Verification items for the finished model (mm, model axes). A direction names the side the tool comes from. Give positions to 0.01 mm unless a question says otherwise; leave off trailing zeros. Write each loop counter-clockwise with the first axis right and the second up, starting at its lowest first coordinate (ties: lowest second). Pieces come first, ordered by that corner, then holes. Notation, with made-up numbers: (21.25, 18.5) - (47.25, 18.5) arc R37 cw to (47.25, 56.5) - close; hole circle Ø6 at (55.25, 67.5). An arc over 180 degrees is marked (long way). Answer as a JSON object with one key per item and string values. Group by question number.
Item 1: Sectioned sample at B-B, the plane x = 0.95. Count the separate pieces of the cut face and the enclosed holes in it, and give its area (3 significant figures).
Item 2: Scan lines: line 1 along Y through (x, z) = (2.3, 0); line 2 along Y through (x, z) = (1.9, 16.5); line 3 along Z through (x, y) = (0.3, 16). Record each from-to range of solid material in increasing order. Write a range as [from, to].
Item 3: Tool access check on faces 1 (the face through (1, -17.1, -15)), 2 (the face through (1, -25, -23)), 3 (the face through (1, -25, 19)), 4 (the face through (2, 32, -35)). Record the directions out of +Z, -Z, +X, -X, +Y, -Y that give a thin tool (end or side, any length) a straight path to the whole face; none if there is none.
Item 4: Sectioned sample at C-C, the plane y = -7.5. Record the boundary of the cut face in (x, z).
Item 5: Sectioned sample at A-A, the plane y = 16. Record the boundary of the cut face in (x, z).
Item 6: Sectioned sample at D-D, the plane z = -20. Record the boundary of the cut face in (x, y).
Item 7: Go/stop test with flat-tipped pins: pin 1 (2 mm diameter, centred on y = -20.5, z = -46.5, fed in from -X); pin 2 (1.5 mm diameter, centred on x = 1.5, z = 16, fed in from -Y); pin 3 (1.5 mm diameter, centred on x = 1.5, y = -16, fed in from -Z); pin 4 (0.9 mm diameter, centred on x = 2, y = 31.5, fed in from -Z). Record where each tip stops, or that it passes through.
Item 8: Draft check along Y on faces 5 (the face through (1.52, 26.39, -36.15)), 6 (the face through (1, 17.1, 15)), 7 (the face through (1.479, -2.609, -59.864)), 8 (the face through (1.5, 15.5, -9.9)). Enter one of: +Y half, -Y half, draft (parallel to the pull), parting line (faces both ways), or undercut.
```python
from build123d import *

# Parameters (mm, degrees)
SKETCH1_R           = 2.1
BOSS_EXTRUDE2_DEPTH = 3
SKETCH2_R           = 7.5
BOSS_EXTRUDE3_DEPTH = 3
SKETCH3_W           = 60
SKETCH3_H           = 10
SKETCH3_R           = 2.6
BOSS_EXTRUDE4_DEPTH = 3
FILLET3_R           = 5
SKETCH4_R           = 1.6
CUT_EXTRUDE1_DEPTH  = 4
FILLET4_R           = 6


with BuildPart() as part:
    # Sketch1 → Boss-Extrude2 (new body)
    with BuildSketch(Plane(origin=(0, 0, 0), x_dir=(0, 0, -1), z_dir=(1, 0, 0))):
        with BuildLine():
            ThreePointArc((35, -25), (60, 0), (35, 25))
            Line((35, 25), (-25, 25))
            Line((-25, 25), (-25, -25))
            Line((-25, -25), (35, -25))
        make_face()
        with BuildLine():
            Line((-11.5, -17.1), (-17.5, -17.1))
            ThreePointArc((-17.5, -17.1), (-19.1, -15.5), (-17.5, -13.9))
            Line((-17.5, -13.9), (-11.5, -13.9))
            ThreePointArc((-11.5, -13.9), (-9.9, -15.5), (-11.5, -17.1))
        make_face(mode=Mode.SUBTRACT)
        with Locations((35, 0)):
            Circle(SKETCH1_R, mode=Mode.SUBTRACT)
        with BuildLine():
            Line((11.5, 17.1), (17.5, 17.1))
            ThreePointArc((17.5, 17.1), (19.1, 15.5), (17.5, 13.9))
            Line((17.5, 13.9), (11.5, 13.9))
            ThreePointArc((11.5, 13.9), (9.9, 15.5), (11.5, 17.1))
        make_face(mode=Mode.SUBTRACT)
        with BuildLine():
            ThreePointArc((4, 11.5), (15.5, 0), (4, -11.5))
            Line((4, -11.5), (-2, -11.5))
            ThreePointArc((-2, -11.5), (-13.5, 0), (-2, 11.5))
            Line((-2, 11.5), (4, 11.5))
        make_face(mode=Mode.SUBTRACT)
        with BuildLine():
            Line((11.5, -13.9), (17.5, -13.9))
            ThreePointArc((17.5, -13.9), (19.1, -15.5), (17.5, -17.1))
            Line((17.5, -17.1), (11.5, -17.1))
            ThreePointArc((11.5, -17.1), (9.9, -15.5), (11.5, -13.9))
        make_face(mode=Mode.SUBTRACT)
        with BuildLine():
            ThreePointArc((-17.5, 13.9), (-19.1, 15.5), (-17.5, 17.1))
            Line((-17.5, 17.1), (-11.5, 17.1))
            ThreePointArc((-11.5, 17.1), (-9.9, 15.5), (-11.5, 13.9))
            Line((-11.5, 13.9), (-17.5, 13.9))
        make_face(mode=Mode.SUBTRACT)
    extrude(amount=BOSS_EXTRUDE2_DEPTH)

    # Sketch2 → Boss-Extrude3 (add)
    with BuildSketch(Plane(origin=(3, 0, 0), x_dir=(0, 0, -1), z_dir=(1, 0, 0))):
        with Locations((0, -24.979991994)):
            Circle(SKETCH2_R)
    extrude(amount=-BOSS_EXTRUDE3_DEPTH)

    # Sketch3 → Boss-Extrude4 (add)
    with BuildSketch(Plane(origin=(3, 0, 0), x_dir=(0, 0, -1), z_dir=(1, 0, 0))):
        with Locations((5, 30)):
            Rectangle(SKETCH3_W, SKETCH3_H)
        with Locations((-16.105832267, 30)):
            Circle(SKETCH3_R, mode=Mode.SUBTRACT)
        with Locations((26.356099555, 30)):
            Circle(SKETCH3_R, mode=Mode.SUBTRACT)
    extrude(amount=-BOSS_EXTRUDE4_DEPTH)

    # Fillet3
    fillet3_edges = [part.edges().sort_by_distance(p)[0] for p in [
        (1.5, 25, -35),
    ]]
    fillet(fillet3_edges, radius=FILLET3_R)

    # Sketch4 → Cut-Extrude1 (cut, through all)
    with BuildSketch(Plane.ZY):
        with Locations((0, -24.979991994)):
            Circle(SKETCH4_R)
    extrude(amount=-CUT_EXTRUDE1_DEPTH, mode=Mode.SUBTRACT)

    # Fillet4
    fillet4_edges = [part.edges().sort_by_distance(p)[0] for p in [
        (1.5, -25, 7.499973312),
        (1.5, -25, -7.499973312),
    ]]
    fillet(fillet4_edges, radius=FILLET4_R)


solid = part.part
```
Geometry check:
{
 "1": {"separate pieces": "1", "enclosed holes": "9", "area": "3,950 mm^2"},
 "2": {"line 1": "[-32.48, -26.58], [-23.38, -11.5], [11.5, 35]", "line 2": "[-25, -17.1], [-13.9, 13.9], [17.1, 27.43], [32.57, 35]", "line 3": "[-54.21, -19.02], [-9.98, 9.98], [19.02, 25]"},
 "3": {"face 1": "+X, -X", "face 2": "-Z, +X, -X, -Y", "face 3": "+Z, +X, -X, -Y", "face 4": "-Z, +X, -X, +Y"},
 "4": {"outline": "(0, -58.85) - (3, -58.85) - (3, -12.72) - (0, -12.72) - close; (0, 10.72) - (3, 10.72) - (3, 25) - (0, 25) - close"},
 "5": {"outline": "(0, -54.21) - (3, -54.21) - (3, -19.02) - (0, -19.02) - close; (0, -9.98) - (3, -9.98) - (3, 9.98) - (0, 9.98) - close; (0, 19.02) - (3, 19.02) - (3, 25) - (0, 25) - close"},
 "6": {"outline": "(0, -25) - (3, -25) - (3, 35) - (0, 35) - close"},
 "7": {"pin 1": "x = 0", "pin 2": "y = -25", "pin 3": "z = -54.81", "pin 4": "z = -35"},
 "8": {"face 5": "+Y half", "face 6": "undercut", "face 7": "parting line", "face 8": "undercut"}
}
